For this review, take the finished solid that the model builds, in its own axes (mm). A direction names the side the tool comes from. Give positions to 0.01 mm unless a question says otherwise; leave off trailing zeros. Loops run counter-clockwise (first coordinate to the right, second up) from the corner with the lowest first, then second, coordinate; pieces in that order, holes last.
```python
from build123d import *

# Parameters (mm, degrees)
BOSS_EXTRUDE1_DEPTH      = 6
BOSS_EXTRUDE1_DEPTH_BACK = 6
FILLET1_R                = 2
SKETCH3_R                = 1.85
CUT_EXTRUDE2_DEPTH       = 4.826
CUT_EXTRUDE2_DEPTH_BACK  = 4.826
SKETCH4_R                = 2.794
CUT_EXTRUDE3_DEPTH       = 4.826


with BuildPart() as part:
    # Sketch1 → Boss-Extrude1 (new body, two sides)
    with BuildSketch(Plane.XY) as boss_extrude1_sk:
        with BuildLine():
            Line((25.8064, 0), (25.8064, 4.826))
            Line((25.8064, 4.826), (20.361415325, 4.826))
            ThreePointArc((20.361415325, 4.826), (0, 18.0174), (-20.361415325, 4.826))
            Line((-20.361415325, 4.826), (-25.8064, 4.826))
            Line((-25.8064, 4.826), (-25.8064, 0))
            Line((-25.8064, 0), (-17.995098923, 0))
            ThreePointArc((-17.995098923, 0), (0, 14.2074), (17.995098923, 0))
            Line((17.995098923, 0), (25.8064, 0))
        make_face()
    extrude(amount=BOSS_EXTRUDE1_DEPTH)
    extrude(boss_extrude1_sk.sketch, amount=-BOSS_EXTRUDE1_DEPTH_BACK)

    # Fillet1
    fillet1_edges = [part.edges().sort_by_distance(p)[0] for p in [
        (20.361415325, 4.826, 0),
        (-20.361415325, 4.826, 0),
    ]]
    fillet(fillet1_edges, radius=FILLET1_R)

    # Sketch3 → Cut-Extrude2 (cut, two sides)
    with BuildSketch(Plane(origin=(0, 0, 0), x_dir=(1, 0, 0), z_dir=(0, 1, 0))) as cut_extrude2_sk:
        with Locations((21.5, 0)):
            Circle(SKETCH3_R)
        with Locations((-21.5, 0)):
            Circle(SKETCH3_R)
    extrude(amount=CUT_EXTRUDE2_DEPTH, mode=Mode.SUBTRACT)
    extrude(cut_extrude2_sk.sketch, amount=-CUT_EXTRUDE2_DEPTH_BACK, mode=Mode.SUBTRACT)

    # Sketch4 → Cut-Extrude3 (cut)
    with BuildSketch(Plane(origin=(0, 4.826, 0), x_dir=(1, 0, 0), z_dir=(0, 1, 0))):
        with Locations((-21.5, 0)):
            Circle(SKETCH4_R)
        with Locations((21.5, 0)):
            Circle(SKETCH4_R)
    extrude(amount=CUT_EXTRUDE3_DEPTH, mode=Mode.SUBTRACT)


solid = part.part
```
Item 1: Tool access review of faces 5 (the flat face through (-24, 4.826, 0)), 6 (the flat face through (24, 4.826, 0)), 7 (the cylindrical face through (0.342, 18.015, 0.084)): name each direction out of +Z, -Z, +X, -X, +Y, -Y from which nothing blocks a thin tool from reaching the whole face with its end or side.
Answer:
face 5: -X, +Y
face 6: +X, +Y
face 7: +Z, -Z, +Y
Item 2: For L1, parallel to Z at x = 21.5, y = 3.05; L2, parallel to X at y = 1.1, z = 0; L3, parallel to X at y = 1.25, z = -0.5, list the stretches that pass through material, from the lowest coordinate up.
Answer:
L1: z = -6 to -1.85, 1.85 to 6
L2: x = -25.81 to -23.35, -19.65 to -17.7, 17.7 to 19.65, 23.35 to 25.81
L3: x = -25.81 to -23.28, -19.72 to -17.65, 17.65 to 19.72, 23.28 to 25.81
Item 3: Clearance check with flat-ended pins moving along their axes: pin 1 Ø4.5 at (x, z) = (21.5, 0) entering from +Y; pin 2 Ø3.5 at (x, z) = (21, 2.5) entering from +Y; pin 3 Ø3 at (x, z) = (-21.5, 0) entering from +Y; pin 4 Ø5 at (y, z) = (13, 4) entering from -X. State where each tip first meets the part, or that it passes through.
Answer:
pin 1: stops at y = 4.83
pin 2: stops at y = 6.98
pin 3: passes through
pin 4: stops at x = -16.7
Item 4: Take a section at C-C on z = 3.75. Give the boundary of the cut face in (x, y), and give its area (3 significant figures).
Answer:
outline: (-25.81, 0) - (-18, 0) arc R18.5 cw to (18, 0) - (25.81, 0) - (25.81, 4.83) - (21.62, 4.83) arc R2 cw to (19.84, 5.91) arc R22.31 ccw to (-19.84, 5.91) arc R2 cw to (-21.62, 4.83) - (-25.81, 4.83) - close
area: 256 mm2
Item 5: Take a section at B-B on y = 9.75. Give the boundary of the cut face in (x, z), and give its area (3 significant figures).
Answer:
outline: (-17.34, -6) - (-12.04, -6) - (-12.04, 6) - (-17.34, 6) - close; (12.04, -6) - (17.34, -6) - (17.34, 6) - (12.04, 6) - close
area: 127 mm2
Item 6: The part is to be moulded in two halves that separate along Z. For faces 1 (the cylindrical face through (20.56, 5.13, 4.15)), 2 (the cylindrical face through (-18.707, 5.987, 0.063)), 3 (the flat face through (-0.1, 14.4, 6)), 4 (the cylindrical face through (19.65, 2.38, -0.08)), say which applies: released by +Z, released by -Z, zero draft, split by the parting line, or undercut.
Answer:
face 1: zero draft
face 2: undercut
face 3: released by +Z
face 4: undercut
Item 7: Take a section at A-A on z = 0. Give the boundary of the cut face in (x, y).
Answer:
outline: (-25.81, 0) - (-23.35, 0) - (-23.35, 4.83) - (-25.81, 4.83) - close; (-19.65, 0) - (-18, 0) arc R18.5 cw to (18, 0) - (19.65, 0) - (19.65, 4.83) - (18.71, 4.83) - (18.71, 7.87) arc R22.31 ccw to (-18.71, 7.87) - (-18.71, 4.83) - (-19.65, 4.83) - close; (23.35, 0) - (25.81, 0) - (25.81, 4.83) - (23.35, 4.83) - close
Item 8: Take a section at D-D on x = -15. Give the boundary of the cut face in (y, z), and give its area (3 significant figures).
Answer:
outline: (6.54, -6) - (12.22, -6) - (12.22, 6) - (6.54, 6) - close
area: 68.2 mm2
